Geometry check sheet. Reference: the model listing, model coordinates, mm. A direction names the side the tool comes from. Round coordinates to 2 decimals unless told otherwise and drop trailing zeros. Write each loop counter-clockwise with the first axis right and the second up, starting at its lowest first coordinate (ties: lowest second). Pieces come first, ordered by that corner, then holes. Notation, with made-up numbers: M -6,45 L 30,45 A21 ccw 30,74 Z; hole C 71,-40 d4. An arc over 180 degrees is marked long. Answer as CSV lines item,"result". Start each with the question number.
```python
from build123d import *

# Parameters (mm, degrees)
F0_W           = 91.8
F0_H           = 73.3
F0_W_2         = 77.3
F0_H_2         = 67.8
F1_DEPTH       = 1.75
F2_DEPTH       = 3.75
F3_D           = 2.7
F3_CSINK_D     = 4.7
F3_CSINK_ANGLE = 90


with BuildPart() as f1:
    # F0 (on Top) → F1 (new body)
    with BuildSketch(Plane.XY):
        with Locations((-1.1, -1.25)):
            Rectangle(F0_W, F0_H)
        with Locations((-1.1, -1.25)):
            Rectangle(F0_W_2, F0_H_2, mode=Mode.SUBTRACT)
    extrude(amount=-F1_DEPTH)

    # F0 (on Top) → F2 (join)
    with BuildSketch(Plane.XY):
        with Locations((-1.1, -1.25)):
            Rectangle(F0_W_2, F0_H_2)
    extrude(amount=-F2_DEPTH)

    # F3 (through all)
    with Locations(Plane.XY):
        with Locations((-44.15, -1.25), (41.75, -1.25)):
            CounterSinkHole(F3_D / 2, F3_CSINK_D / 2, counter_sink_angle=F3_CSINK_ANGLE)


solid = f1.part
```
1) Section check B-B, the plane y = -1.25. Record the cut outline in (x, z).
2) Access from +Z, -Z, +X, -X, +Y, -Y to the whole of each face (thin tool, end or side, straight path). Record for faces 4 (the flat face through (37.55, -2, -3)), 5 (the flat face through (-39.75, -2, -3)), 6 (the flat face through (-2, -1, 0)), 7 (the cylindrical face through (43.1, -1.2, -1.4)), 8 (the flat face through (-2, 32.65, -3)).
3) Section check C-C, the plane y = -26.5. Record the cut outline in (x, z), plus the area to 3 significant figures.
4) Mould release check, pull along Y, two halves, no side actions. Record for faces 1 (the flat face through (-2, -35.15, -3)), 2 (the cylindrical face through (-45.397, -1.767, -1.38)), 3 (the flat face through (-2, -1, -3.75)): released by +Y, released by -Y, zero draft, split by the parting line, or undercut.
5) Section check A-A, the plane x = 41.75. Record the cut outline in (y, z), plus the area to 3 significant figures.
6) Scan lines: line 1 (X direction, y = -1, z = -1.4); line 2 (Y direction, x = -44.15, z = -1.25); line 3 (X direction, y = 7, z = -3.6). Record each from-to range of solid material in increasing order. Write a range as from..to.
7) Go/stop test with flat-tipped pins: pin 1 (2.5 mm diameter, centred on x = 41.75, y = -1.25, fed in from -Z); pin 2 (1 mm diameter, centred on x = 1.5, z = -3, fed in from +Y); pin 3 (0.6 mm diameter, centred on y = 12.5, z = -3, fed in from -X); pin 4 (2 mm diameter, centred on x = 12, z = -3, fed in from -Y). Record where each tip stops, or that it passes through.
8) Section check D-D, the plane x = -33.5. Record the cut outline in (y, z), plus the area to 3 significant figures.
Results:
1,outline,"M -47,-1.75 L -45.5,-1.75 L -45.5,-1 L -46.5,0 L -47,0 Z; M -42.8,-1.75 L -39.75,-1.75 L -39.75,-3.75 L 37.55,-3.75 L 37.55,-1.75 L 40.4,-1.75 L 40.4,-1 L 39.4,0 L -41.8,0 L -42.8,-1 Z; M 43.1,-1.75 L 44.8,-1.75 L 44.8,0 L 44.1,0 L 43.1,-1 Z"
2,face 4,"-Z, +X, +Y, -Y"
2,face 5,"-Z, -X, +Y, -Y"
2,face 6,"+Z, +X, -X, +Y, -Y"
2,face 7,"+Z, -Z"
2,face 8,"-Z, +X, -X, +Y"
3,outline,"M -47,-1.75 L -39.75,-1.75 L -39.75,-3.75 L 37.55,-3.75 L 37.55,-1.75 L 44.8,-1.75 L 44.8,0 L -47,0 Z"
3,area,"315 mm^2"
4,face 1,"released by -Y"
4,face 2,"undercut"
4,face 3,"zero draft"
5,outline,"M -37.9,-1.75 L -2.6,-1.75 L -2.6,-1 L -3.6,0 L -37.9,0 Z; M 0.1,-1.75 L 35.4,-1.75 L 35.4,0 L 1.1,0 L 0.1,-1 Z"
5,area,"123 mm^2"
6,line 1,"x = -47..-45.48, -42.82..40.42, 43.08..44.8"
6,line 2,"y = -37.9..-2.6, 0.1..35.4"
6,line 3,"x = -39.75..37.55"
7,pin 1,"passes through"
7,pin 2,"stops at y = 32.65"
7,pin 3,"stops at x = -39.75"
7,pin 4,"stops at y = -35.15"
8,outline,"M -37.9,-1.75 L -35.15,-1.75 L -35.15,-3.75 L 32.65,-3.75 L 32.65,-1.75 L 35.4,-1.75 L 35.4,0 L -37.9,0 Z"
8,area,"264 mm^2"
